from build123d import *

# Parameters (mm, degrees)
F1_DEPTH = 5
F3_DEPTH = 20
F5_DEPTH = 20.001
F7_D     = 7.23
F9_DEPTH = 5.001
F10_D    = 5.5
F11_D    = 5.5


with BuildPart() as f1:
    # F0 (on Top) → F1 (new body)
    with BuildSketch(Plane.XY):
        Polygon((33, 0), (0, 0), (0, -60), (33, -60), (33, -45), (33, -15), align=None)
    extrude(amount=F1_DEPTH)

    # F2 (on face) → F3 (join)
    with BuildSketch(Plane.XY.offset(5)):
        Polygon((0, -20), (20, -20), (20, 0), (15, 0), (15, -15), (5, -15), (5, 0), (0, 0), align=None)
        Polygon((20, -40), (0, -40), (0, -60), (5, -60), (5, -45), (15, -45), (15, -60), (20, -60), align=None)
    extrude(amount=F3_DEPTH)

    # F4 (on face) → F5 (cut, through all)
    with BuildSketch(Plane.YZ.offset(20)):
        Polygon((0, 25), (-20, 25), (0, 5), align=None)
        Polygon((-60, 5), (-40, 25), (-60, 25), align=None)
    extrude(amount=-F5_DEPTH, mode=Mode.SUBTRACT)

    # F7 (through all)
    with Locations(Plane(origin=(0, 0, 0), x_dir=(1, 0, 0), z_dir=(0, 0, -1))):
        with Locations((26.5, 7.5), (26.5, 52.5)):
            Hole(F7_D / 2)

    # F8 (on face) → F9 (cut, through all)
    with BuildSketch(Plane.XY.offset(5)):
        Polygon((31, -39.2240850911), (31, -20.7759149089), (22, -30), align=None)
        Polygon((22, -27.136144826), (31, -17.912059735), (22, -21.3735981965), align=None)
        Polygon((22, -32.863855174), (22, -38.6264018035), (31, -42.087940265), align=None)
    extrude(amount=-F9_DEPTH, mode=Mode.SUBTRACT)

    # F10 (through all)
    with Locations(Plane(origin=(0, 0, 0), x_dir=(1, 0, 0), z_dir=(0, 0, -1))):
        with Locations((10, 30)):
            Hole(F10_D / 2)

    # F11 (through all)
    with Locations(Plane.XZ.offset(45)):
        with Locations((10, 15)):
            Hole(F11_D / 2)


solid = f1.part
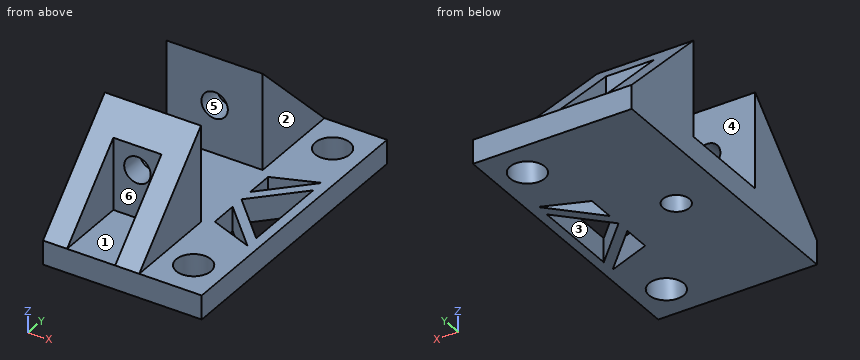
The model under review builds one solid part; all positions refer to its coordinate system, in mm. Face numbers are marked on the shaded views. A direction names the side the tool comes from. Round coordinates to 2 decimals unless told otherwise and drop trailing zeros. Loops run counter-clockwise (first coordinate to the right, second up) from the corner with the lowest first, then second, coordinate; pieces in that order, holes last. Notation, with made-up numbers: (-4, 83) -> (15, 83) arc R25 ccw to (15, 112) -> close; hole circle Ø6 at (-18.75, 22). An arc over 180 degrees is marked (long way). Write item = value, one per line. Start each with the question number.
Item 1: Take a section at A-A on y = -7.5. Give the boundary of the cut face in (x, z) (3 decimals).
Item 2: For the marked faces 1, 2 and 3, list the 3-axis set-ups (+Z, -Z, +X, -X, +Y, -Y) from which the entire face can be reached by the end or side of a thin tool; tool diameter is ignored.
Item 3: Take a section at C-C on x = 10. Give the boundary of the cut face in (y, z).
Item 4: Mouldability with a two-part tool opening along Y and no side actions: class the marked faces 4, 5 and 6 as released by +Y, released by -Y, zero draft, split by the parting line, or undercut.
Item 5: Take a section at D-D on z = 7. Give the boundary of the cut face in (x, y), plus the area to 3 significant figures.
Item 6: Take a section at B-B on z = 3.75. Give the boundary of the cut face in (x, y) (3 decimals).
Item 7: Insertion check: pin 1 (8 mm diameter, centred on x = 19, z = 12, fed in from -Y); pin 2 (1.5 mm diameter, centred on x = 11.5, z = 6, fed in from +Y); pin 3 (8 mm diameter, centred on x = 10.5, y = -50, fed in from +Z). Each pin has a flat end and moves straight along its axis. Give the tip position at first contact, or say it passes through.
Item 8: To check wall thickness, follow L1, parallel to Y at x = 2, z = 20; L2, parallel to X at y = -52.5, z = 1.6 (3 decimals); L3, parallel to Y at x = 26.5, z = 3.25 (3 decimals). State the ranges of each line that lie inside material, in increasing order.
Result:
q1.outline = (0, 0) -> (22.885, 0) -> (22.885, 5) -> (20, 5) -> (20, 12.5) -> (15, 12.5) -> (15, 5) -> (5, 5) -> (5, 12.5) -> (0, 12.5) -> close; (30.115, 0) -> (33, 0) -> (33, 5) -> (30.115, 5) -> close
q2.face_1 = +Z, -Y
q2.face_2 = +Z, +X, +Y, -Y
q2.face_3 = +Z, -Z
q3.outline = (-60, 0) -> (-32.75, 0) -> (-32.75, 5) -> (-40, 5) -> (-40, 12.25) -> (-45, 12.25) -> (-45, 5) -> (-60, 5) -> close; (-45, 17.75) -> (-40, 17.75) -> (-40, 25) -> (-45, 20) -> close; (-27.25, 0) -> (0, 0) -> (0, 5) -> (-15, 5) -> (-15, 12.25) -> (-20, 12.25) -> (-20, 5) -> (-27.25, 5) -> close; (-20, 17.75) -> (-15, 17.75) -> (-15, 20) -> (-20, 25) -> close
q4.face_4 = undercut
q4.face_5 = zero draft
q4.face_6 = released by -Y
q5.outline = (0, -58) -> (5, -58) -> (5, -45) -> (15, -45) -> (15, -58) -> (20, -58) -> (20, -40) -> (0, -40) -> close; (0, -20) -> (20, -20) -> (20, -2) -> (15, -2) -> (15, -15) -> (5, -15) -> (5, -2) -> (0, -2) -> close
q5.area = 460 mm²
q6.outline = (0, -60) -> (33, -60) -> (33, 0) -> (0, 0) -> close; hole circle Ø5.5 at (10, -30); hole (22, -38.626) -> (31, -42.088) -> (22, -32.864) -> close; hole (22, -30) -> (31, -39.224) -> (31, -20.776) -> close; hole (22, -27.136) -> (31, -17.912) -> (22, -21.374) -> close; hole circle Ø7.23 at (26.5, -52.5); hole circle Ø7.23 at (26.5, -7.5)
q7.pin_1 = -57
q7.pin_2 = -15
q7.pin_3 = 5
q8.L1 = -45 to -40, -20 to -15
q8.L2 = 0 to 22.885, 30.115 to 33
q8.L3 = -60 to -56.115, -48.885 to -40.357, -37.476 to -34.612, -25.388 to -22.524, -19.643 to -11.115, -3.885 to 0
